Build history of the part. All positions in model axes, mm. Round coordinates to 2 decimals unless told otherwise and drop trailing zeros. Write each loop counter-clockwise with the first axis right and the second up, starting at its lowest first coordinate (ties: lowest second). Pieces come first, ordered by that corner, then holes. Notation, with made-up numbers: (87.25, -16.5) -> (100.25, -16.5) arc R29 ccw to (100.25, 4.5) -> close; hole circle Ø3 at (-24, 53). An arc over 180 degrees is marked (long way). Return JSON: item names as keys, results as strings.
Autodesk Inventor part; units mm, degrees
ref_plane "Work Plane1" through (0, 0, 577.85) normal (0, 0, -1) x (-1, 0, 0)
ref_plane "YZ Plane" through (0, 0, 0) normal (1, 0, 0) x (0, 1, 0)
ref_plane "XZ Plane" through (0, 0, 0) normal (0, 1, 0) x (-1, 0, 0)
sketch "Sketch1" plane through (0, 0, 0) normal (0, 0, 1) x (1, 0, 0)
  circle A0 centre (0, 0) radius 31.75
  dimension "d0" = 63.5
extrude "Extrusion1" add sketch "Sketch1" along normal blind 1155.7
sketch "Sketch2" plane through (0, 0, 0) normal (0, 0, -1) x (-1, 0, 0)
  circle A0 centre (0, 0) radius 9.525
  dimension "d3" = 19.05
extrude "Extrusion2" add sketch "Sketch2" along normal blind 50.8
sketch "Sketch3" plane through (0, 0, 0) normal (0, 1, 0) x (-1, 0, 0)
  circle A0 centre (0, -63.5) radius 33.02
  line L0 (31.75, 0) -> (-31.75, 0)
  point P0 (0, 0)
  dimension "d6" = 63.5
  dimension "d7" = 66.04
extrude "Extrusion3" add sketch "Sketch3" along normal mid plane 19.05
ref_plane "Work Plane1" through (0, 0, 577.85) normal (0, 0, -1) x (-1, 0, 0)
mirror "Mirror1" about plane through (0, 0, 577.85) normal (0, 0, -1) of "Extrusion3", "Extrusion2"
properties part number "driveshaft_m_mount_shaft"
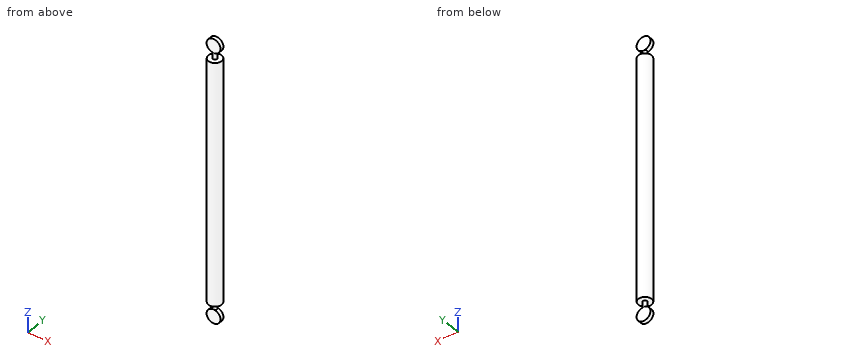
Q1. Pin check, flat tips, straight feed: pin 1 Ø6 at (x, y) = (0.5, 15) entering from +Z; pin 2 Ø6 at (x, y) = (10.5, -5.5) entering from +Z; pin 3 Ø6 at (x, z) = (-2, 1063) entering from +Y. Stop position of each tip, or through.
Verdict:
{"pin 1": "stops at z = 1155.7", "pin 2": "stops at z = 1251.36", "pin 3": "stops at y = 31.75"}
Q2. Saw through at B-B on x = -19.5. List the corners of the cut face in (y, z) (3 decimals), then the cut area to 3 significant figures.
Verdict:
{"outline": "(-25.056, 0) -> (25.056, 0) -> (25.056, 1155.7) -> (-25.056, 1155.7) -> close; (-9.525, -90.147) -> (9.525, -90.147) -> (9.525, -36.853) -> (-9.525, -36.853) -> close; (-9.525, 1192.553) -> (9.525, 1192.553) -> (9.525, 1245.847) -> (-9.525, 1245.847) -> close", "area": "59,900 mm²"}
Q3. Saw through at A-A on y = 0. List the corners of the cut face in (x, z) (3 decimals).
Verdict:
{"outline": "(-31.75, 0) -> (-9.525, 0) -> (-9.525, -31.884) arc R33.02 ccw (long way) to (9.525, -31.884) -> (9.525, 0) -> (31.75, 0) -> (31.75, 1155.7) -> (9.525, 1155.7) -> (9.525, 1187.584) arc R33.02 ccw (long way) to (-9.525, 1187.584) -> (-9.525, 1155.7) -> (-31.75, 1155.7) -> close"}
Q4. Wall check: L1, parallel to Z at x = 27.5, y = 4.5; L2, parallel to Z at x = 24, y = 8; L3, parallel to Z at x = -19.5, y = -19.5. Give the ranges that are in metal, low to high.
Verdict:
{"L1": "z = -81.78 to -45.22, 0 to 1155.7, 1200.92 to 1237.48", "L2": "z = -86.18 to -40.82, 0 to 1155.7, 1196.52 to 1241.88", "L3": "z = 0 to 1155.7"}
Q5. Saw through at C-C on z = 971. List the corners of the cut face in (x, y), then the cut area to 3 significant figures.
Verdict:
{"outline": "circle Ø63.5 at (0, 0)", "area": "3,170 mm²"}
